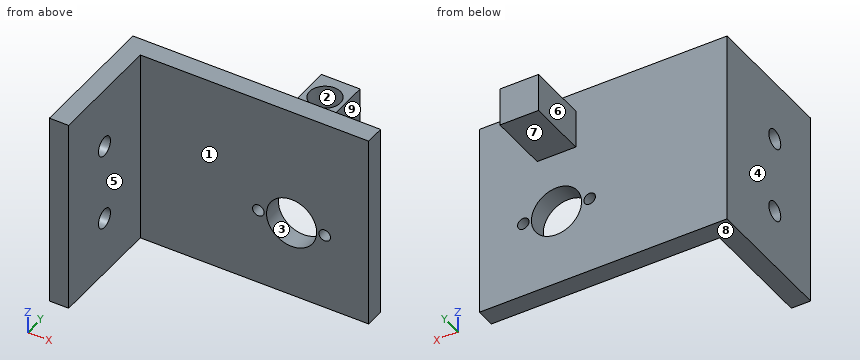
```python
from build123d import *

# Parameters (mm, degrees)
SKETCH3_W           = 40
SKETCH3_H           = 50.8
BOSS_EXTRUDE1_DEPTH = 5
SKETCH4_W           = 10
SKETCH4_H           = 10
BOSS_EXTRUDE2_DEPTH = 15.6
SKETCH5_R           = 4
CUT_EXTRUDE4_DEPTH  = 8
SKETCH6_W           = 50.8
SKETCH6_H           = 5
BOSS_EXTRUDE3_DEPTH = 24.225
SKETCH8_W           = 5
SKETCH8_H           = 50.8
BOSS_EXTRUDE4_DEPTH = 30
SKETCH9_R           = 2.5
CUT_EXTRUDE5_DEPTH  = 5
SKETCH10_R          = 6.5
SKETCH10_R_2        = 1.5
CUT_EXTRUDE6_DEPTH  = 5


with BuildPart() as part:
    # Sketch3 → Boss-Extrude1 (new body)
    with BuildSketch(Plane(origin=(0, 0, 0), x_dir=(1, 0, 0), z_dir=(0, 1, 0))):
        with Locations((0, -5.4)):
            Rectangle(SKETCH3_W, SKETCH3_H)
    extrude(amount=BOSS_EXTRUDE1_DEPTH)

    # Sketch4 → Boss-Extrude2 (add)
    with BuildSketch(Plane(origin=(0, 5, 0), x_dir=(1, 0, 0), z_dir=(0, 1, 0))):
        with Locations((0, -20.8)):
            Rectangle(SKETCH4_W, SKETCH4_H)
    extrude(amount=BOSS_EXTRUDE2_DEPTH)

    # Sketch5 → Cut-Extrude4 (cut)
    with BuildSketch(Plane.XY.offset(25.8)):
        with Locations((0, 14)):
            Circle(SKETCH5_R)
    extrude(amount=-CUT_EXTRUDE4_DEPTH, mode=Mode.SUBTRACT)

    # Sketch6 → Boss-Extrude3 (add)
    with BuildSketch(Plane.ZY.offset(20)):
        with Locations((5.4, 2.5)):
            Rectangle(SKETCH6_W, SKETCH6_H)
    extrude(amount=BOSS_EXTRUDE3_DEPTH)

    # Sketch8 → Boss-Extrude4 (add)
    with BuildSketch(Plane.XZ):
        with Locations((-41.725, 5.4)):
            Rectangle(SKETCH8_W, SKETCH8_H)
    extrude(amount=BOSS_EXTRUDE4_DEPTH)

    # Sketch9 → Cut-Extrude5 (cut)
    with BuildSketch(Plane.ZY.offset(44.225)):
        with Locations((-4.8, -15)):
            Circle(SKETCH9_R)
        with Locations((15.2, -15)):
            Circle(SKETCH9_R)
    extrude(amount=-CUT_EXTRUDE5_DEPTH, mode=Mode.SUBTRACT)

    # Sketch10 → Cut-Extrude6 (cut)
    with BuildSketch(Plane(origin=(0, 5, 0), x_dir=(1, 0, 0), z_dir=(0, 1, 0))):
        with Locations(Location((0, 0, 0), (0, 0, 270))):
            Circle(SKETCH10_R)
        with Locations(Location((-8.6, 0, 0), (0, 0, 270))):
            Circle(SKETCH10_R_2)
        with Locations(Location((8.6, 0, 0), (0, 0, 270))):
            Circle(SKETCH10_R_2)
    extrude(amount=-CUT_EXTRUDE6_DEPTH, mode=Mode.SUBTRACT)


solid = part.part
```
Check sheet for the modelled part. Datum: model origin and axes. Units: mm. Face numbers are marked on the shaded views. A direction names the side the tool comes from. Coordinates: 2 decimals unless noted, no trailing zeros. Order: outer loops, then holes, each group sorted by start corner. A loop starts at its lowest first (then second) coordinate and runs counter-clockwise, first axis right, second up. Notation, with made-up numbers: (72.25, 19.5) -> (110.25, 19.5) arc R16 ccw to (110.25, 31.5) -> close; hole circle Ø1 at (56.5, 88). An arc over 180 degrees is marked (long way). Write each question's results on one line, items separated by ' | '. Start each with the question number.
1) Material ranges on line 1 along Y through (x, z) = (0, 22.5); line 2 along Y through (x, z) = (-41.05, 15.2); line 3 along Y through (x, z) = (10, 2.5), recorded low to high.
2) Draft check along X on the marked faces 1, 2, 3 and 4. Enter one of: pulls with the +X half, pulls with the -X half, needs draft (parallel to the pull), parting line crosses it, or undercut.
3) Section check D-D (y = 14). Enter the section's corners in (x, z), and give its area (3 significant figures).
4) Section check B-B (x = -8.6). Enter the section's corners in (y, z).
5) Section check A-A (z = 0). Enter the section's corners in (x, y) (3 decimals).
6) Set-up check for the marked faces 5, 6, 7, 8 and 9: record each of +Z, -Z, +X, -X, +Y, -Y from which the full face is reachable in a straight line by a thin tool's end or side.
7) Depth check by flat-ended pin: pin 1 (8 mm diameter, centred on x = 2.5, z = 4.5, fed in from +Y); pin 2 (5 mm diameter, centred on x = -8.6, z = 0, fed in from -Y); pin 3 (8 mm diameter, centred on x = 0, z = 0, fed in from +Y); pin 4 (11 mm diameter, centred on x = -2.5, y = 9, fed in from -Z). Enter the tip coordinate at first touch or a pass-through.
8) Section check C-C (y = -15). Enter the section's corners in (x, z) (3 decimals), and give its area (3 significant figures).
Checked values:
1) line 1: 0 to 10, 18 to 20.6 | line 2: -30 to -17.5, -12.5 to 5 | line 3: 0 to 5
2) face 1: needs draft | face 2: undercut | face 3: undercut | face 4: pulls with the -X half
3) outline: (-5, 15.8) -> (5, 15.8) -> (5, 25.8) -> (4, 25.8) -> (4, 17.8) -> (-4, 17.8) -> (-4, 25.8) -> (-5, 25.8) -> close | area: 36.0 mm²
4) outline: (0, -20) -> (5, -20) -> (5, -1.5) -> (0, -1.5) -> close; (0, 1.5) -> (5, 1.5) -> (5, 30.8) -> (0, 30.8) -> close
5) outline: (-44.225, -30) -> (-39.225, -30) -> (-39.225, 0) -> (-10.1, 0) -> (-10.1, 5) -> (-44.225, 5) -> close; (-7.1, 0) -> (-6.5, 0) -> (-6.5, 5) -> (-7.1, 5) -> close; (6.5, 0) -> (7.1, 0) -> (7.1, 5) -> (6.5, 5) -> close; (10.1, 0) -> (20, 0) -> (20, 5) -> (10.1, 5) -> close
6) face 5: +Z, -Z, +X, -Y | face 6: +Z, -Z, -X, +Y | face 7: -Z, +X, -X, +Y | face 8: -Z, +X, -X, +Y, -Y | face 9: +Z, -Z, +X, +Y
7) pin 1: y = 5 | pin 2: y = 0 | pin 3: through | pin 4: z = -20
8) outline: (-44.225, -20) -> (-39.225, -20) -> (-39.225, -7.3) -> (-44.225, -7.3) -> close; (-44.225, -2.3) -> (-39.225, -2.3) -> (-39.225, 12.7) -> (-44.225, 12.7) -> close; (-44.225, 17.7) -> (-39.225, 17.7) -> (-39.225, 30.8) -> (-44.225, 30.8) -> close | area: 204 mm²
